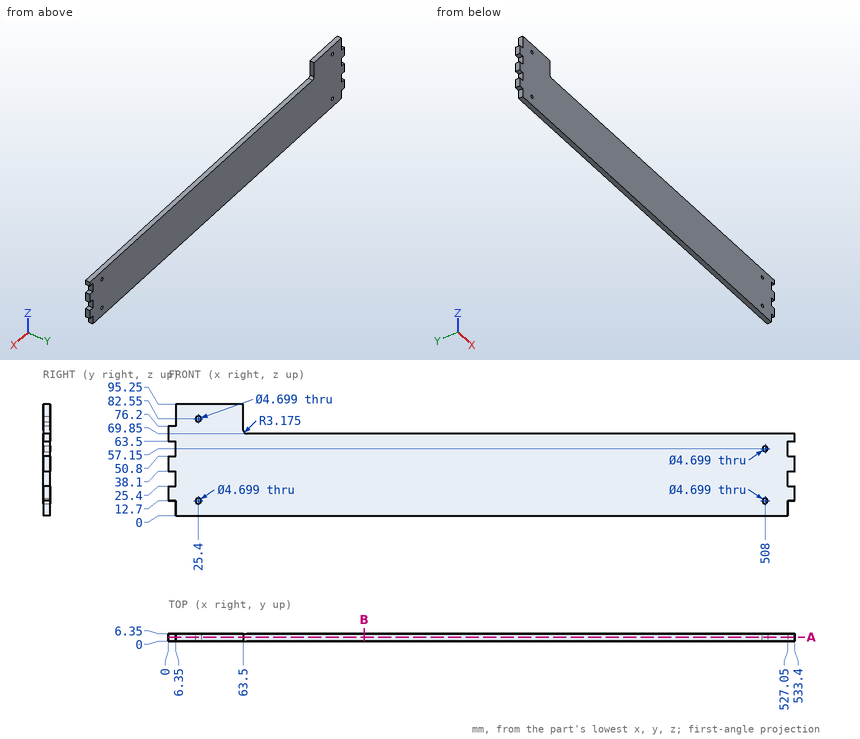
Job drawing, mm, ordinate dimensions from the low corner. One solid piece. Give positions to 0.01 mm unless a question says otherwise; leave off trailing zeros. Loops run counter-clockwise (first coordinate to the right, second up) from the corner with the lowest first, then second, coordinate; pieces in that order, holes last. Notation, with made-up numbers: M 56,29.25 L 105,29.25 A4 cw 105,36.25 Z; hole C -17,-19 d3. An arc over 180 degrees is marked long. Answer in a Markdown table with one row per item. Add a question column.
Item 1: Drop flat-ended pins along their axis: P1, Ø3, axis at x = 4.5, y = 4.5, coming from the -Z side; P2, Ø3, axis at x = 528.5, y = 2.5, coming from the +Z side; P3, Ø1.9, axis at y = 3.5, z = 58, coming from the -X side. Give the stop position or say it passes through.
Item 2: Band-saw the part on A-A on y = 3.5. Give the number of separate pieces and of enclosed holes in the cut face, then the cut area to 3 significant figures.
Item 3: Band-saw the part on B-B on x = 166.5. Give the cut face in (y, z).
Item 4: Probe probe 1 along Z at (x, y) = (25.4, 4); probe 2 along Z at (x, y) = (508, 3); probe 3 along Z at (x, y) = (401, 6). List the from-to ranges inside material, lowest first.
Reply:
| question | item | result |
|---|---|---|
| 1 | P1 | stops at z = 12.7 |
| 1 | P2 | stops at z = 69.85 |
| 1 | P3 | stops at x = 6.35 |
| 2 | separate pieces | 1 |
| 2 | enclosed holes | 4 |
| 2 | area | 38,200 mm^2 |
| 3 | outline | M 0,0 L 6.35,0 L 6.35,69.85 L 0,69.85 Z |
| 4 | probe 1 | z = 0 to 10.35, 15.05 to 80.2, 84.9 to 95.25 |
| 4 | probe 2 | z = 0 to 10.35, 15.05 to 54.8, 59.5 to 69.85 |
| 4 | probe 3 | z = 0 to 69.85 |
